For this review, take the finished solid that the model builds, in its own axes (mm). A direction names the side the tool comes from. Coordinates: 2 decimals unless noted, no trailing zeros. Write each loop counter-clockwise with the first axis right and the second up, starting at its lowest first coordinate (ties: lowest second). Pieces come first, ordered by that corner, then holes. Notation, with made-up numbers: (-30.5, 56) -> (19.5, 56) arc R18 cw to (19.5, 67) -> close; hole circle Ø10 at (46.25, -8). An arc over 180 degrees is marked (long way). Put each result on its own line as item: value. Start each with the question number.
Item 1: Insertion check: P1, Ø10, axis at x = 0, y = 0, coming from the -Z side; P2, Ø12, axis at y = -9, z = -6, coming from the +X side; P3, Ø10, axis at y = -3.5, z = -9.5, coming from the +X side; P4, Ø1.6, axis at x = 0.5, y = -16, coming from the +Z side. Each pin has a flat end and moves straight along its axis. Give the tip position at first contact, or say it passes through.
Item 2: Consider section B-B on z = -17.25. Give the boundary of the cut face in (x, y), and give its area (3 significant figures).
Item 3: To check wall thickness, follow L1, parallel to Z at x = 6, y = 10.5; L2, parallel to Z at x = 8, y = -2; L3, parallel to Y at x = 1, z = -7.5. State the ranges of each line that lie inside material, in increasing order.
Item 4: Consider section C-C on x = 2. Give the number of separate pieces and of enclosed holes in the cut face, and give its area (3 significant figures).
Item 5: For faces 1 (the flat face through (4.3, -11.81, -15.23)), 2 (the cylindrical face through (-6.91, 4.03, -15.33)), 3 (the flat face through (-0.25, 8, -5)), 4 (the flat face through (-4.254, -11.687, -15.227)), list the 3-axis set-ups (+Z, -Z, +X, -X, +Y, -Y) from which the entire face can be reached by the end or side of a thin tool; tool diameter is ignored.
Item 6: Consider section A-A on y = 0. Give the boundary of the cut face in (x, z).
Item 7: The part is to be moulded in two halves that separate along Z. For faces 5 (the cylindrical face through (6.87, 8.88, -5.03)), 6 (the flat face through (-7.994, 9.527, -15.227)), 7 (the flat face through (-3, -3, -10.3)), say which applies: +Z half, -Z half, draft (parallel to the pull), parting line (faces both ways), or undercut.
Autodesk Inventor part; units mm, degrees
ref_plane "KUPPLUNG_XY" through (0, 0, 0) normal (0, 0, 1) x (1, 0, 0)
ref_plane "KUPPLUNG_YZ" through (0, 0, 0) normal (1, 0, 0) x (0, 1, 0)
ref_plane "KUPPLUNG_ZX" through (0, 0, 0) normal (0, 1, 0) x (0, 0, 1)
sketch "Sketch_1" plane through (0, 0, 0) normal (1, 0, 0) x (0, 1, 0)
  line L0 (0, -10.3) -> (0, 0)
  line L1 (0, 0) -> (15.5, 0)
  line L2 (15.5, 0) -> (16, -0.5)
  line L3 (16, -0.5) -> (16, -10.3)
  line L4 (16, -10.3) -> (0, -10.3)
  line L5 (0, -10.3) -> (0, 0)
revolve "Revolution1" add sketch "Sketch_1" angle 360 about axis through (0, 0, -10.3) along (0, 0, -1)
sketch "Sketch_2" plane through (0, 0, -10.1) normal (0, 0, 1) x (1, 0, 0)
  line L0 (-16.7417, 2.952) -> (-7.8785, 1.3892)
  arc A0 (-5.1423, 6.1284) -> (-7.8785, 1.3892) centre (0, 0) ccw
  line L1 (-5.1423, 6.1284) -> (-10.9274, 13.0228)
  arc A1 (-10.9274, 13.0228) -> (-16.7417, 2.952) centre (0, 0) ccw
extrude "Extrusion1" add sketch "Sketch_2" against normal blind 10.4
sketch "Sketch_3" plane through (0, 0, -10.1) normal (0, 0, 1) x (1, 0, 0)
  arc A0 (-5.8143, -15.9748) -> (5.8143, -15.9748) centre (0, 0) ccw
  line L0 (5.8143, -15.9748) -> (2.7362, -7.5175)
  arc A1 (-2.7362, -7.5175) -> (2.7362, -7.5175) centre (0, 0) ccw
  line L1 (-2.7362, -7.5175) -> (-5.8143, -15.9748)
extrude "Extrusion2" add sketch "Sketch_3" against normal blind 10.4
sketch "Sketch_19" plane through (0, 0, -10.1) normal (0, 0, 1) x (1, 0, 0)
  arc A0 (7.8785, 1.3892) -> (5.1423, 6.1284) centre (0, 0) ccw
  line L0 (7.8785, 1.3892) -> (16.7417, 2.952)
  arc A1 (16.7417, 2.952) -> (10.9274, 13.0228) centre (0, 0) ccw
  line L1 (10.9274, 13.0228) -> (5.1423, 6.1284)
extrude "Extrusion3" add sketch "Sketch_19" against normal blind 10.4
sketch "Sketch_9" plane through (0, 0, 0) normal (1, 0, 0) x (0, 1, 0)
  line L0 (0, -28.3636) -> (0, 0)
  line L1 (0, 0) -> (3, 0)
  line L2 (3, 0) -> (3, -5.5091)
  line L3 (3, -5.5091) -> (3.8727, -5.5091)
  line L4 (3.8727, -5.5091) -> (3.8727, -11.8909)
  line L5 (3.8727, -11.8909) -> (2.4545, -11.8909)
  line L6 (2.4545, -11.8909) -> (2.4545, -13.2545)
  line L7 (2.4545, -13.2545) -> (1.1275, -13.2545)
  line L8 (1.1275, -13.2545) -> (1.1275, -28.1275)
  line L9 (1.1275, -28.1275) -> (1.3636, -28.3636)
  line L10 (1.3636, -28.3636) -> (0, -28.3636)
  line L11 (0, -28.3636) -> (0, 0)
  dimension "d36" = 3
revolve "Revolution3" cut sketch "Sketch_9" angle 360 about axis through (0, 0, -28.3636) along (0, 0, -1)
sketch "Sketch_12" plane through (0, 0, 0) normal (0, 0, 1) x (1, 0, 0)
  line L0 (-0.25, 16) -> (-0.25, 0)
  line L1 (-0.25, 0) -> (0.25, 0)
  line L2 (0.25, 0) -> (0.25, 16)
  line L3 (0.25, 16) -> (-0.25, 16)
extrude "Extrusion10" cut sketch "Sketch_12" against normal blind 10.1
sketch "Sketch_13" plane through (0, 0, -5.1) normal (0, 0, 1) x (1, 0, 0)
  line L0 (13.5, 10.5) -> (-16.5, 10.5)
  line L1 (-16.5, 10.5) -> (-16.5, 14.1)
  line L2 (-16.5, 14.1) -> (-4.5, 14.1)
  line L3 (-4.5, 14.1) -> (-4.5, 12.5)
  line L4 (-4.5, 12.5) -> (-4.121, 12.121)
  line L5 (-4.121, 12.121) -> (13.5, 12.121)
  line L6 (13.5, 12.121) -> (13.5, 10.5)
  line L7 (13.5, 10.5) -> (-16.5, 10.5)
revolve "Revolution6" cut sketch "Sketch_13" angle 360 about axis through (13.5, 10.5, -5.1) along (-1, 0, 0)
thread "Thread2"
sketch "Sketch_11" plane through (0, 0, -21.8) normal (0, 0, 1) x (0, 1, 0)
  arc A0 (-1.8674, -0.5726) -> (-1.4296, -1.3309) centre (-1.5586, -0.8998) ccw
  arc A1 (-0.4378, -1.9035) -> (-1.4296, -1.3309) centre (-1.2039, -2.0852) ccw
  arc A2 (-0.4378, -1.9035) -> (0.4378, -1.9035) centre (0, -1.7997) ccw
  arc A3 (1.4296, -1.3309) -> (0.4378, -1.9035) centre (1.2039, -2.0852) ccw
  arc A4 (1.4296, -1.3309) -> (1.8674, -0.5726) centre (1.5586, -0.8998) ccw
  arc A5 (1.8674, 0.5726) -> (1.8674, -0.5726) centre (2.4078, 0) ccw
  arc A6 (1.8674, 0.5726) -> (1.4296, 1.3309) centre (1.5586, 0.8999) ccw
  arc A7 (0.4378, 1.9035) -> (1.4296, 1.3309) centre (1.2039, 2.0852) ccw
  arc A8 (0.4378, 1.9035) -> (-0.4378, 1.9035) centre (0, 1.7997) ccw
  arc A9 (-1.4296, 1.3309) -> (-0.4378, 1.9035) centre (-1.2039, 2.0852) ccw
  arc A10 (-1.4296, 1.3309) -> (-1.8674, 0.5726) centre (-1.5586, 0.8999) ccw
  arc A11 (-1.8674, -0.5726) -> (-1.8674, 0.5726) centre (-2.4078, 0) ccw
extrude "Extrusion11" cut sketch "Sketch_11" against normal blind 2.64
sketch "Sketch_15" plane through (-8.5, 10.5, -5.1) normal (-1, 0, 0) x (0, 1, 0)
  arc A0 (-1.6394, -0.5027) -> (-1.2551, -1.1684) centre (-1.3683, -0.79) ccw
  arc A1 (-0.3843, -1.6711) -> (-1.2551, -1.1684) centre (-1.0569, -1.8307) ccw
  arc A2 (-0.3843, -1.6711) -> (0.3843, -1.6711) centre (0, -1.58) ccw
  arc A3 (1.2551, -1.1684) -> (0.3843, -1.6711) centre (1.0569, -1.8307) ccw
  arc A4 (1.2551, -1.1684) -> (1.6394, -0.5027) centre (1.3683, -0.79) ccw
  arc A5 (1.6394, 0.5027) -> (1.6394, -0.5027) centre (2.1139, 0) ccw
  arc A6 (1.6394, 0.5027) -> (1.2551, 1.1684) centre (1.3683, 0.79) ccw
  arc A7 (0.3843, 1.6711) -> (1.2551, 1.1684) centre (1.0569, 1.8307) ccw
  arc A8 (0.3843, 1.6711) -> (-0.3843, 1.6711) centre (0, 1.58) ccw
  arc A9 (-1.2551, 1.1684) -> (-0.3843, 1.6711) centre (-1.0569, 1.8307) ccw
  arc A10 (-1.2551, 1.1684) -> (-1.6394, 0.5027) centre (-1.3683, 0.79) ccw
  arc A11 (-1.6394, -0.5027) -> (-1.6394, 0.5027) centre (-2.1139, 0) ccw
extrude "Extrusion12" cut sketch "Sketch_15" against normal blind 2.34
ref_plane "KUPPLUNG_XY" through (0, 0, 0) normal (0, 0, 1) x (1, 0, 0)
ref_plane "KUPPLUNG_YZ" through (0, 0, 0) normal (1, 0, 0) x (0, 1, 0)
ref_plane "KUPPLUNG_ZX" through (0, 0, 0) normal (0, 1, 0) x (0, 0, 1)
properties part number "Coupling"
Return value:
1. P1: z = -10.3
1. P2: x = 15.72
1. P3: x = 16
1. P4: z = 0
2. outline: (-16.74, 2.95) -> (-7.88, 1.39) arc R8 cw to (-5.14, 6.13) -> (-10.93, 13.02) arc R17 ccw to start; (-5.81, -15.97) arc R17 ccw to (5.81, -15.97) -> (2.74, -7.52) arc R8 cw to (-2.74, -7.52) -> close; (5.14, 6.13) arc R8 cw to (7.88, 1.39) -> (16.74, 2.95) arc R17 ccw to (10.93, 13.02) -> close
2. area: 236 mm^2
3. L1: -10.3 to -6.72, -3.48 to 0
3. L2: -10.3 to 0
3. L3: -15.97 to -3.74, 3.74 to 15.97
4. separate pieces: 2
4. enclosed holes: 1
4. area: 355 mm^2
5. face 1: -Z, +X
5. face 2: -Z
5. face 3: +Z, +Y
5. face 4: -Z, -X
6. outline: (-16, -10.3) -> (-3.87, -10.3) -> (-3.87, -5.51) -> (-3, -5.51) -> (-3, 0) -> (-15.5, 0) -> (-16, -0.5) -> close; (3, -5.51) -> (3.87, -5.51) -> (3.87, -10.3) -> (16, -10.3) -> (16, -0.5) -> (15.5, 0) -> (3, 0) -> close
7. face 5: undercut
7. face 6: draft
7. face 7: -Z half
